Design review of the part built by this model. Coordinates are the model's own, in mm. Face numbers are marked on the shaded views. Give positions to 0.01 mm unless a question says otherwise; leave off trailing zeros. Write each loop counter-clockwise with the first axis right and the second up, starting at its lowest first coordinate (ties: lowest second). Pieces come first, ordered by that corner, then holes. Notation, with made-up numbers: M 58.25,44.5 L 74.25,44.5 A21 cw 74.25,55.5 Z; hole C -40,76.5 d11. An arc over 180 degrees is marked long. Write each question's results on one line, items separated by ' | '. Start each with the question number.
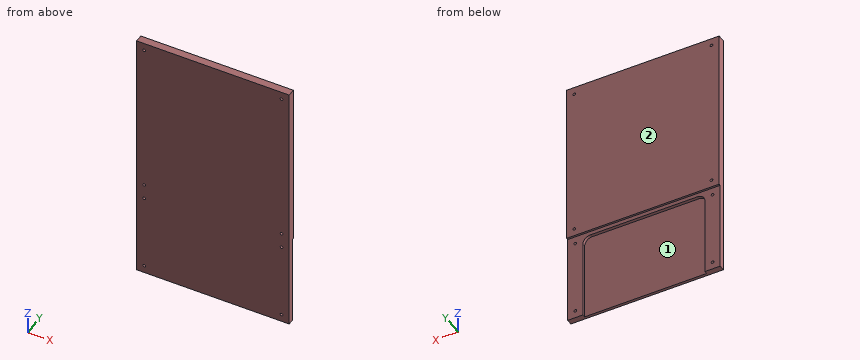
from build123d import *

# Parameters (mm, degrees)
SKETCH1_W                   = 127
SKETCH1_H                   = 215.9
BOSS_EXTRUDE1_DEPTH         = 6.35
SKETCH3_W                   = 127
SKETCH3_H                   = 76.2
CUT_EXTRUDE1_DEPTH          = 1.5875
F_43_0_089_DIAMETER_HOLE1_D = 2.2606
F_43_0_089_DIAMETER_HOLE2_D = 2.2606
SKETCH8_W                   = 101.6
SKETCH8_H                   = 73.025
CUT_EXTRUDE2_DEPTH          = 2.54
FILLET1_R                   = 6.35


with BuildPart() as part:
    # Sketch1 → Boss-Extrude1 (new body)
    with BuildSketch(Plane(origin=(0, 0, 0), x_dir=(1, 0, 0), z_dir=(0, 1, 0))):
        with Locations((63.5, 107.95)):
            Rectangle(SKETCH1_W, SKETCH1_H)
    extrude(amount=BOSS_EXTRUDE1_DEPTH)

    # Sketch3 → Cut-Extrude1 (cut)
    with BuildSketch(Plane(origin=(0, 6.35, 0), x_dir=(1, 0, 0), z_dir=(0, 1, 0))):
        with Locations((63.5, 177.8)):
            Rectangle(SKETCH3_W, SKETCH3_H)
    extrude(amount=-CUT_EXTRUDE1_DEPTH, mode=Mode.SUBTRACT)

    # #43 (0.089) Diameter Hole1 (through all)
    with Locations(Plane(origin=(0, 4.7625, 0), x_dir=(1, 0, 0), z_dir=(0, 1, 0))):
        with Locations((6.35, 209.55), (6.35, 146.05), (120.65, 146.05), (120.65, 209.55)):
            Hole(F_43_0_089_DIAMETER_HOLE1_D / 2)

    # #43 (0.089) Diameter Hole2 (through all)
    with Locations(Plane(origin=(0, 6.35, 0), x_dir=(1, 0, 0), z_dir=(0, 1, 0))):
        with Locations((6.35, 6.35), (120.65, 6.35), (6.35, 133.35), (120.65, 133.35)):
            Hole(F_43_0_089_DIAMETER_HOLE2_D / 2)

    # Sketch8 → Cut-Extrude2 (cut)
    with BuildSketch(Plane(origin=(0, 4.7625, 0), x_dir=(1, 0, 0), z_dir=(0, 1, 0))):
        with Locations((63.5, 179.3875)):
            Rectangle(SKETCH8_W, SKETCH8_H)
    extrude(amount=-CUT_EXTRUDE2_DEPTH, mode=Mode.SUBTRACT)

    # Fillet1
    fillet1_edges = [part.edges().sort_by_distance(p)[0] for p in [
        (12.7, 3.4925, -142.875),
        (114.3, 3.4925, -142.875),
    ]]
    fillet(fillet1_edges, radius=FILLET1_R)


solid = part.part
Q1. We need section C-C on z = -161. Write out the cut boundary in (x, y).
Q2. The part is to be moulded in two halves that separate along X. For the marked faces 1 and 2, say which applies: pulls with the +X half, pulls with the -X half, needs draft (parallel to the pull), parting line crosses it, or undercut.
Q3. Wall thickness on line 1 along X through (y, z) = (4, -133.35); line 2 along Z through (x, y) = (120.65, 2.75); line 3 along X through (y, z) = (3.5, -189): over which ranges is each line inside the solid? List them lowest first. Write a range as from..to.
Q4. For pin 1 Ø2.5 at (x, z) = (120.65, -146.05) entering from +Y; pin 2 Ø1.5 at (x, z) = (43, -170) entering from +Y; pin 3 Ø1.8 at (x, z) = (120.65, -209.55) entering from +Y; pin 4 Ø1.7 at (x, y) = (39, 5.5) entering from -Z (3 decimals), all flat-tipped, find the tip position at first contact; note any pin that passes through.
Q5. We need section A-A on y = 3.25. Count the separate pieces of the cut face and the enclosed holes in it, and give its area (3 significant figures).
Answer sheet:
1) outline: M 0,0 L 127,0 L 127,4.76 L 114.3,4.76 L 114.3,2.22 L 12.7,2.22 L 12.7,4.76 L 0,4.76 Z
2) face 1: undercut | face 2: needs draft
3) line 1: 0..5.22, 7.48..119.52, 121.78..127 | line 2: -215.9..-210.68, -208.42..-147.18, -144.92..-134.48, -132.22..-7.48, -5.22..0 | line 3: 0..12.7, 114.3..127
4) pin 1: y = 4.76 | pin 2: y = 2.22 | pin 3: through | pin 4: z = -142.875
5) separate pieces: 1 | enclosed holes: 8 | area: 20,000 mm^2
